Geometry: final body of the model. Coordinates: model frame, mm. Face numbers are marked on the shaded views. A direction names the side the tool comes from. Round coordinates to 2 decimals unless told otherwise and drop trailing zeros. Order: outer loops, then holes, each group sorted by start corner. A loop starts at its lowest first (then second) coordinate and runs counter-clockwise, first axis right, second up. Notation, with made-up numbers: (23.25, -16.5) - (58.25, -16.5) arc R24 ccw to (58.25, 22.5) - close; hole circle Ø4 at (-15, -26). An arc over 180 degrees is marked (long way). Put each result on its own line as item: value. Start each with the question number.
(1) Section A-A (z = 25). Output: boundary loops of the cut face in (x, y).
(2) Section D-D (x = 101.6). Output: boundary loops of the cut face in (y, z).
(3) Pin query (flat end, axial travel): P1, Ø8, axis at y = -17.5, z = 118.5, coming from the +X side; P2, Ø12, axis at x = 110, y = -41.5, coming from the +Z side; P3, Ø12.5, axis at x = 65, y = -13.5, coming from the -Z side. Return the tip coordinate at first contact, or that it passes through.
(4) Pull-direction query (X, two-part tool) for the marked faces 4, 5 and 6; classes: released by +X, released by -X, zero draft, split by the parting line, or undercut.
(5) Section B-B (y = -30.5). Output: boundary loops of the cut face in (x, z) (3 decimals), and give its area (3 significant figures).
(6) Access query for the marked faces 1, 2 and 3. Directions: +Z, -Z, +X, -X, +Y, -Y. A direction counts if a zero-diameter tool reaches every point of the face in a straight line with its end or side. Return the directions, or none.
(7) Section C-C (z = 46). Output: boundary loops of the cut face in (x, y).
(8) Material intervals for L1, parallel to X at y = -42, z = 46; L2, parallel to X at y = -43.5, z = 53.5; L3, parallel to X at y = -13, z = 34.5, sorted ascending. Write a range as [from, to].
from build123d import *

# Parameters (mm, degrees)
F1_DEPTH = 50.8


with BuildPart() as f1:
    # F0 (on Front) → F1 (new body)
    with BuildSketch(Plane.XZ):
        with BuildLine():
            Line((0, 123.825), (0, 0))
            Line((0, 0), (31.75, 0))
            Line((31.75, 0), (31.75, 60.325))
            Line((31.75, 60.325), (50.8, 60.325))
            Line((50.8, 60.325), (50.8, 35.57891))
            Line((50.8, 35.57891), (76.2, 35.57891))
            ThreePointArc((76.2, 35.57891), (101.6, 60.97891), (127, 35.57891))
            Line((127, 35.57891), (127, 10.17891))
            Line((127, 10.17891), (152.4, 10.17891))
            Line((152.4, 10.17891), (152.4, 107.95))
            Line((152.4, 107.95), (95.25, 107.95))
            Line((95.25, 107.95), (95.25, 123.825))
            Line((95.25, 123.825), (88.9, 123.825))
            ThreePointArc((88.9, 123.825), (63.5, 98.425), (38.1, 123.825))
            Line((38.1, 123.825), (0, 123.825))
        make_face()
    extrude(amount=F1_DEPTH)


solid = f1.part
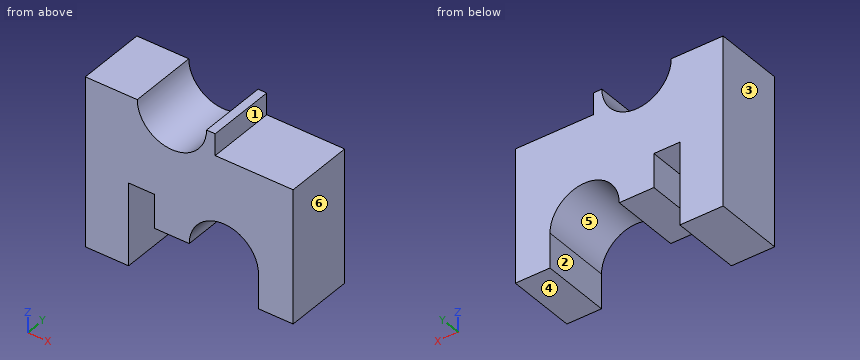
Checks:
1. outline: (0, -50.8) - (31.75, -50.8) - (31.75, 0) - (0, 0) - close; (127, -50.8) - (152.4, -50.8) - (152.4, 0) - (127, 0) - close
2. outline: (-50.8, 60.98) - (0, 60.98) - (0, 107.95) - (-50.8, 107.95) - close
3. P1: stops at x = 95.25
3. P2: stops at z = 107.95
3. P3: stops at z = 35.58
4. face 4: zero draft
4. face 5: undercut
4. face 6: released by +X
5. outline: (0, 0) - (31.75, 0) - (31.75, 60.325) - (50.8, 60.325) - (50.8, 35.579) - (76.2, 35.579) arc R25.4 cw to (127, 35.579) - (127, 10.179) - (152.4, 10.179) - (152.4, 107.95) - (95.25, 107.95) - (95.25, 123.825) - (88.9, 123.825) arc R25.4 cw to (38.1, 123.825) - (0, 123.825) - close
5. area: 11,800 mm²
6. face 1: +Z, +X, +Y, -Y
6. face 2: -Z, +Y, -Y
6. face 3: +Z, -Z, -X, +Y, -Y
7. outline: (0, -50.8) - (31.75, -50.8) - (31.75, 0) - (0, 0) - close; (50.8, -50.8) - (78.44, -50.8) - (78.44, 0) - (50.8, 0) - close; (124.76, -50.8) - (152.4, -50.8) - (152.4, 0) - (124.76, 0) - close
8. L1: x = [0, 31.75], [50.8, 78.44], [124.76, 152.4]
8. L2: x = [0, 31.75], [50.8, 83.6], [119.6, 152.4]
8. L3: x = [0, 31.75], [127, 152.4]
